from build123d import *

# Parameters (mm, degrees)
SKETCH2_W                       = 25
SKETCH2_H                       = 130
SKETCH2_R                       = 5.1
SKETCH2_R_2                     = 7.5
BOSS_EXTRUDE1_DEPTH             = 6.35
TAP_DRILL_FOR_M3X0_5_TAP1_D     = 2.5
TAP_DRILL_FOR_M3X0_5_TAP1_DEPTH = 12.5
TAP_DRILL_FOR_M3X0_5_TAP1_TIP   = 0.751075774
BOSS_EXTRUDE2_DEPTH             = 6.35
F_1_4_CLEARANCE_HOLE1_D         = 6.7564
TAP_DRILL_FOR_M3X0_5_TAP2_D     = 2.5
M3_CLEARANCE_HOLE1_OUTLINE_R    = 1.7
M3_CLEARANCE_HOLE1_DEPTH        = 6.35


# Read off the part's stored shape, not the designer's step: M3 Clearance Hole1
with BuildPart() as part:
    # Sketch2 → Boss-Extrude1 (new body)
    with BuildSketch(Plane.XY):
        with Locations((0, 43.85)):
            Rectangle(SKETCH2_W, SKETCH2_H)
        Circle(SKETCH2_R, mode=Mode.SUBTRACT)
        with Locations((0, 25)):
            Circle(SKETCH2_R_2, mode=Mode.SUBTRACT)
        with Locations((0, 50)):
            Circle(SKETCH2_R_2, mode=Mode.SUBTRACT)
    extrude(amount=BOSS_EXTRUDE1_DEPTH)

    # Tap Drill for M3x0.5 Tap1
    with Locations(Plane.ZY.offset(12.5)):
        with Locations((3.175, 50), (3.175, 0), (3.175, 25)):
            Hole(TAP_DRILL_FOR_M3X0_5_TAP1_D / 2, depth=TAP_DRILL_FOR_M3X0_5_TAP1_DEPTH)
            with Locations((0, 0, -(TAP_DRILL_FOR_M3X0_5_TAP1_DEPTH + TAP_DRILL_FOR_M3X0_5_TAP1_TIP / 2))):  # 118° drill point
                Cone(0, TAP_DRILL_FOR_M3X0_5_TAP1_D / 2, TAP_DRILL_FOR_M3X0_5_TAP1_TIP, mode=Mode.SUBTRACT)

    # Sketch8 → Boss-Extrude2 (add)
    with BuildSketch(Plane(origin=(0, 0, 0), x_dir=(-1, 0, 0), z_dir=(0, 0, -1))):
        Polygon((12.5, 73.85), (22.5, 83.85), (22.5, 108.85), (12.5, 108.85), align=None)
    extrude(amount=-BOSS_EXTRUDE2_DEPTH)

    # 1/4 Clearance Hole1 (through all)
    with Locations(Plane.XY.offset(6.35)):
        with Locations((-12.5, 86.85), (-12.5, 100.85)):
            Hole(F_1_4_CLEARANCE_HOLE1_D / 2)

    # Tap Drill for M3x0.5 Tap2 (through all)
    with Locations(Plane.XY.offset(6.35)):
        with Locations((-8, 0), (0, 8), (8, 0), (0, -8)):
            Hole(TAP_DRILL_FOR_M3X0_5_TAP2_D / 2)

    # M3 Clearance Hole1 outline → M3 Clearance Hole1 (cut)
    with BuildSketch(Plane.XY):
        with Locations((-7.5, -16.15)):
            Circle(M3_CLEARANCE_HOLE1_OUTLINE_R)
    extrude(amount=M3_CLEARANCE_HOLE1_DEPTH, mode=Mode.SUBTRACT)


solid = part.part
Part model, mm, in its own coordinate system. A direction names the side the tool comes from. Give positions to 0.01 mm unless a question says otherwise; leave off trailing zeros. Order: outer loops, then holes, each group sorted by start corner. A loop starts at its lowest first (then second) coordinate and runs counter-clockwise, first axis right, second up. Notation, with made-up numbers: (76.5, 47.5) - (92.5, 47.5) arc R16 ccw to (92.5, 77.5) - close; hole circle Ø11 at (15, -20). An arc over 180 degrees is marked (long way). Use a Markdown table: item, result.
1) Probe L1, parallel to Y at x = -7.5, z = 3.25; L2, parallel to X at y = 30.5, z = 3.5; L3, parallel to Y at x = 4, z = 1. List the from-to ranges inside material, lowest first. Write a range as from..to.
Checked values:
| item | result |
|---|---|
| L1 | -21.15..-17.85, -14.45..-1.25, 1.25..23.75, 26.25..48.75, 51.25..108.85 |
| L2 | -12.5..-5.1, 5.1..12.5 |
| L3 | -21.15..-3.16, 3.16..18.66, 31.34..43.66, 56.34..108.85 |
2) Saw through at A-A on y = -16.15. List the corners of the cut face in (x, z).
Checked values:
| item | result |
|---|---|
| outline | (-12.5, 0) - (-9.2, 0) - (-9.2, 6.35) - (-12.5, 6.35) - close; (-5.8, 0) - (12.5, 0) - (12.5, 6.35) - (-5.8, 6.35) - close |
3) Saw through at C-C on y = 50. List the corners of the cut face in (x, z) (3 decimals).
Checked values:
| item | result |
|---|---|
| outline | (-12.5, 0) - (-7.5, 0) - (-7.5, 1.925) - (-12.5, 1.925) - close; (-12.5, 4.425) - (-7.5, 4.425) - (-7.5, 6.35) - (-12.5, 6.35) - close; (7.5, 0) - (12.5, 0) - (12.5, 6.35) - (7.5, 6.35) - close |
4) Two-plate mould, pull along Z, no slides. Class faces 1 (the flat face through (-1, 59, 6.35)), 2 (the cylindrical face through (-7.87, -17.81, 3.13)), 3 (the cylindrical face through (-10.718, 0.375, 1.983)): +Z half, -Z half, draft (parallel to the pull), parting line (faces both ways), or undercut.
Checked values:
| item | result |
|---|---|
| face 1 | +Z half |
| face 2 | draft |
| face 3 | undercut |
5) Saw through at B-B on x = 0. List the corners of the cut face in (y, z), plus the area to 3 significant figures.
Checked values:
| item | result |
|---|---|
| outline | (-21.15, 0) - (-9.25, 0) - (-9.25, 6.35) - (-21.15, 6.35) - close; (-6.75, 0) - (-5.1, 0) - (-5.1, 6.35) - (-6.75, 6.35) - close; (5.1, 0) - (6.75, 0) - (6.75, 6.35) - (5.1, 6.35) - close; (9.25, 0) - (17.5, 0) - (17.5, 6.35) - (9.25, 6.35) - close; (32.5, 0) - (42.5, 0) - (42.5, 6.35) - (32.5, 6.35) - close; (57.5, 0) - (108.85, 0) - (108.85, 6.35) - (57.5, 6.35) - close |
| area | 538 mm² |
6) 3-axis set-ups, long thin cutter, end or side, ignore diameter. For faces 4 (the cylindrical face through (-6.111, 0.375, 1.983)), 5 (the flat face through (-12.5, 26, 5)), 6 (the cylindrical face through (4.864, 1.532, 3.131)): which of +Z, -Z, +X, -X, +Y, -Y reach the whole face in a straight line?
Checked values:
| item | result |
|---|---|
| face 4 | -X |
| face 5 | +Z, -Z, -X, -Y |
| face 6 | +Z, -Z |
7) Saw through at D-D on y = 0. List the corners of the cut face in (x, z) (3 decimals), plus the area to 3 significant figures.
Checked values:
| item | result |
|---|---|
| outline | (-12.5, 0) - (-9.25, 0) - (-9.25, 1.925) - (-12.5, 1.925) - close; (-12.5, 4.425) - (-9.25, 4.425) - (-9.25, 6.35) - (-12.5, 6.35) - close; (-6.75, 0) - (-5.1, 0) - (-5.1, 1.925) - (-6.75, 1.925) - close; (-6.75, 4.425) - (-5.1, 4.425) - (-5.1, 6.35) - (-6.75, 6.35) - close; (5.1, 0) - (6.75, 0) - (6.75, 6.35) - (5.1, 6.35) - close; (9.25, 0) - (12.5, 0) - (12.5, 6.35) - (9.25, 6.35) - close |
| area | 50.0 mm² |
8) Flat gauge pins, fed straight in: P1, Ø2, axis at y = 25, z = 3.175, coming from the -X side; P2, Ø2, axis at y = 0, z = 3.175, coming from the -X side; P3, Ø3, axis at y = 19.5, z = 3, coming from the -X side. Where does each tip first touch, or does it go through?
Checked values:
| item | result |
|---|---|
| P1 | x = 7.43 |
| P2 | x = 5 |
| P3 | x = -12.5 |
